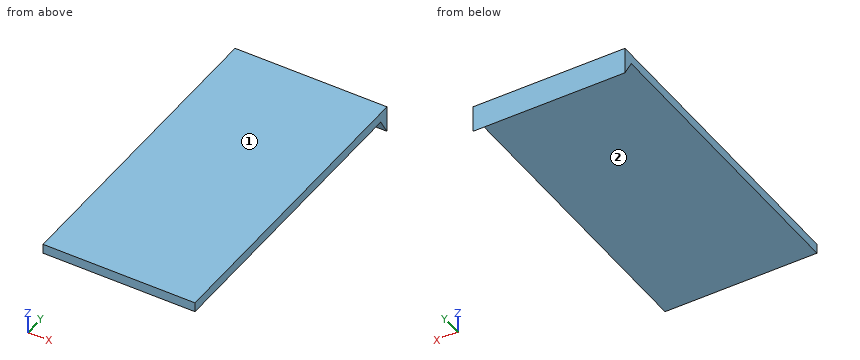
```python
from build123d import *

# Parameters (mm, degrees)
ESQUISSE1_W        = 47
ESQUISSE1_H        = 93.5
BOSS_EXTRU_1_DEPTH = 3
BOSS_EXTRU_2_DEPTH = 47


with BuildPart() as part:
    # Esquisse1 → Boss.-Extru.1 (new body)
    with BuildSketch(Plane.XY):
        with Locations((23.5, 46.75)):
            Rectangle(ESQUISSE1_W, ESQUISSE1_H)
    extrude(amount=-BOSS_EXTRU_1_DEPTH)

    # Esquisse2 → Boss.-Extru.2 (add)
    with BuildSketch(Plane(origin=(47, 0, 0), x_dir=(0, 0, -1), z_dir=(1, 0, 0))):
        Polygon((3, 93.5), (8.284087356, 96.675), (0, 96.675), (0, 93.5), align=None)
    extrude(amount=-BOSS_EXTRU_2_DEPTH)


solid = part.part
```
Could you check a few things on this model? Use its own coordinates, in mm. Face numbers are marked on the shaded views. A direction names the side the tool comes from. Coordinates: 2 decimals unless noted, no trailing zeros. Loops run counter-clockwise (first coordinate to the right, second up) from the corner with the lowest first, then second, coordinate; pieces in that order, holes last. Notation, with made-up numbers: M -30.75,78.25 L 26.25,78.25 A23 cw 26.25,117.25 Z; hole C 78.5,-22.5 d11. An arc over 180 degrees is marked long. Put each result on its own line as item: value. Start each with the question number.
(1) Suppose I cut it at A-A on x = 16.5. Please give me the cut outline in (y, z) (3 decimals).
(2) For the marked faces 1 and 2, which set-ups out of +Z, -Z, +X, -X, +Y, -Y let a thin tool reach every point of the face, with its end or its side?
(3) Will these pins go through, and if not, where does the flat tip stop? P1, Ø5, axis at x = 25.5, y = 15.5, coming from the -Z side; P2, Ø4, axis at x = 33.5, z = -5.5, coming from the -Y side.
(4) I need wall thicknesses on line 1 (Z direction, x = 7, y = 36); line 2 (Y direction, x = 23, z = -7.75) (3 decimals); line 3 (Y direction, x = 34.5, z = -5.5) (3 decimals). Which ranges of each line are inside material? Lowest first, please. Write a range as from..to.
(5) Suppose I cut it at C-C on z = -7. Please give me the cut outline in (x, y) (3 decimals), then the cut area to 3 significant figures.
(6) Suppose I cut it at B-B on y = 90.5. Please give me the cut outline in (x, z).
Solutions:
1. outline: M 0,-3 L 93.5,-3 L 96.675,-8.284 L 96.675,0 L 0,0 Z
2. face 1: +Z, +X, -X, +Y, -Y
2. face 2: -Z, +X, -X, -Y
3. P1: stops at z = -3
3. P2: stops at y = 93.8
4. line 1: z = -3..0
4. line 2: y = 96.354..96.675
4. line 3: y = 95.002..96.675
5. outline: M 0,95.903 L 47,95.903 L 47,96.675 L 0,96.675 Z
5. area: 36.3 mm2
6. outline: M 0,-3 L 47,-3 L 47,0 L 0,0 Z
